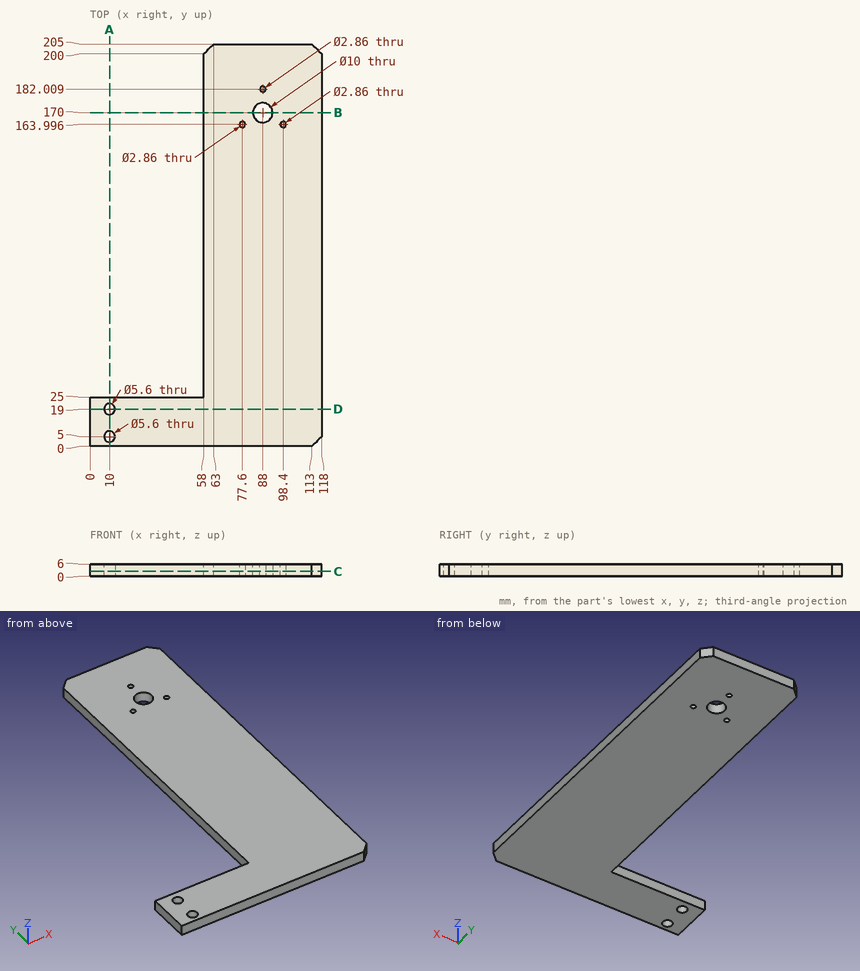
Answer from the drawing. Dimensions are ordinates in mm from the lowest x, y and z of the part. Round coordinates to 2 decimals unless told otherwise and drop trailing zeros. Write each loop counter-clockwise with the first axis right and the second up, starting at its lowest first coordinate (ties: lowest second). Pieces come first, ordered by that corner, then holes. Notation, with made-up numbers: M -9.5,19.25 L 31.5,19.25 A9 cw 31.5,27.25 Z; hole C -31,8.5 d6. An arc over 180 degrees is marked long. Write each question's results on one line, items separated by ' | '. Start each with the question number.
Item 1: Find section D-D on y = 19. Write down the section's boundary in (x, z).
Item 2: Find section A-A on x = 10. Write down the section's boundary in (y, z).
Item 3: Find section B-B on y = 170. Write down the section's boundary in (x, z).
Item 4: Given pin 1 Ø12 at (x, y) = (47.5, 161) entering from +Z; pin 2 Ø2 at (y, z) = (27.5, 0.5) entering from -X; pin 3 Ø3 at (x, z) = (16, 2.5) entering from +Y, each flat-ended and moving along its own axis, determine where each tip first touches the part or whether it passes through.
Item 5: Straight lines are drawn through the part: probe 1 along Y at (x, z) = (10, 3.45); probe 2 along Y at (x, z) = (77.6, 3.8) (1 decimal); probe 3 along Y at (x, z) = (20, 1.4). For each, find the intervals that lie inside material, in ascending order.
Item 6: Find section C-C on z = 2.45. Write down the section's boundary in (x, y) (1 decimal).
Answer block:
1) outline: M 0,0 L 7.2,0 L 7.2,6 L 0,6 Z; M 12.8,0 L 118,0 L 118,6 L 12.8,6 Z
2) outline: M 0,0 L 2.2,0 L 2.2,6 L 0,6 Z; M 7.8,0 L 16.2,0 L 16.2,6 L 7.8,6 Z; M 21.8,0 L 25,0 L 25,6 L 21.8,6 Z
3) outline: M 58,0 L 83,0 L 83,6 L 58,6 Z; M 93,0 L 118,0 L 118,6 L 93,6 Z
4) pin 1: passes through | pin 2: stops at x = 58 | pin 3: stops at y = 25
5) probe 1: y = 0 to 2.2, 7.8 to 16.2, 21.8 to 25 | probe 2: y = 0 to 162.6, 165.4 to 205 | probe 3: y = 0 to 25
6) outline: M 0,0 L 113,0 L 118,5 L 118,200 L 113,205 L 63,205 L 58,200 L 58,25 L 0,25 Z; hole C 10,5 d5.6; hole C 10,19 d5.6; hole C 77.6,164 d2.9; hole C 88,170 d10; hole C 88,182 d2.9; hole C 98.4,164 d2.9
